Geometry: final body of the model. Coordinates: model frame, mm. Face numbers are marked on the shaded views. A direction names the side the tool comes from. Give positions to 0.01 mm unless a question says otherwise; leave off trailing zeros. Write each loop counter-clockwise with the first axis right and the second up, starting at its lowest first coordinate (ties: lowest second). Pieces come first, ordered by that corner, then holes. Notation, with made-up numbers: (-9.75, 10) - (-5.75, 10) arc R6 cw to (-5.75, 15) - close; hole circle Ø1 at (-6.75, -30). An arc over 180 degrees is marked (long way). One line per question, with ' | ' between items. Start each with the question number.
```python
from build123d import *

# Parameters (mm, degrees)
SALIENTE_EXTRUIR1_DEPTH           = 2
SALIENTE_EXTRUIR4_DEPTH           = 28
CROQUIS6_W                        = 6.2
CROQUIS6_H                        = 25
CORTAR_EXTRUIR2_DEPTH             = 6.2
CORTAR_EXTRUIR3_REACH             = 24
CROQUIS7_R                        = 1.6
CORTAR_EXTRUIR4_REACH             = 25.8
CROQUIS8_R                        = 1.6
CORTAR_EXTRUIR5_DEPTH             = 16.8
CORTAR_EXTRUIR6_DEPTH             = 2.5
CORTAR_EXTRUIR6_DIRECTION_2_REACH = 19
CROQUIS11_W                       = 0.3
CROQUIS11_H                       = 13.87
CORTAR_EXTRUIR7_DEPTH             = 6.2
CORTAR_EXTRUIR8_REACH             = 8.5
CROQUIS12_R                       = 1.6
CORTAR_EXTRUIR9_DEPTH             = 3
CORTAR_EXTRUIR10_DEPTH            = 6.5


with BuildPart() as part:
    # Croquis1 → Saliente-Extruir1 (new body)
    with BuildSketch(Plane.XY):
        Polygon((0, 0), (0, -4), (11, -4), (17, -10), (17, -17), (24, -17), (24, 0), (15.5, 0), (9.5, 6), (9.5, 11.13), (6.5, 11.13), (6.5, 25), (0, 25), align=None)
    extrude(amount=SALIENTE_EXTRUIR1_DEPTH)

    # Croquis5 → Saliente-Extruir4 (add)
    with BuildSketch(Plane.XY.offset(2)):
        Polygon((22, -17), (22, -3.5), (24, -3.5), (24, 0), (15.5, 0), (9.5, 6), (9.5, 11.13), (6.5, 11.13), (6.5, 25), (0, 25), (0, -4), (11, -4), (17, -10), (17, -17), align=None)
    extrude(amount=SALIENTE_EXTRUIR4_DEPTH)

    # Croquis6 → Cortar-Extruir2 (cut)
    with BuildSketch(Plane.XY.offset(30)):
        with Locations((3.1, 12.5)):
            Rectangle(CROQUIS6_W, CROQUIS6_H)
    extrude(amount=-CORTAR_EXTRUIR2_DEPTH, mode=Mode.SUBTRACT)

    # Croquis7 → Cortar-Extruir3 (cut, up to next)
    with BuildSketch(Plane(origin=(22, 0, 0), x_dir=(0, 0, -1), z_dir=(1, 0, 0)), mode=Mode.PRIVATE) as cortar_extruir3_sk1:
        with Locations((-18.55, -6.05)):
            Circle(CROQUIS7_R)
    cortar_extruir3_tool1 = extrude(cortar_extruir3_sk1.sketch, amount=-CORTAR_EXTRUIR3_REACH, mode=Mode.PRIVATE) & part.part
    add(cortar_extruir3_tool1.solids().sort_by_distance((22, -6.05, 18.55))[0], mode=Mode.SUBTRACT)
    # Croquis7 → Cortar-Extruir3 (cut, up to next)
    with BuildSketch(Plane(origin=(22, 0, 0), x_dir=(0, 0, -1), z_dir=(1, 0, 0)), mode=Mode.PRIVATE) as cortar_extruir3_sk2:
        with Locations((-6.45, -6.05)):
            Circle(CROQUIS7_R)
    cortar_extruir3_tool2 = extrude(cortar_extruir3_sk2.sketch, amount=-CORTAR_EXTRUIR3_REACH, mode=Mode.PRIVATE) & part.part
    add(cortar_extruir3_tool2.solids().sort_by_distance((22, -6.05, 6.45))[0], mode=Mode.SUBTRACT)

    # Croquis8 → Cortar-Extruir4 (cut, up to next)
    with BuildSketch(Plane.XY.offset(23.8), mode=Mode.PRIVATE) as cortar_extruir4_sk1:
        with Locations((3.1, 4)):
            Circle(CROQUIS8_R)
    cortar_extruir4_tool1 = extrude(cortar_extruir4_sk1.sketch, amount=-CORTAR_EXTRUIR4_REACH, mode=Mode.PRIVATE) & part.part
    add(cortar_extruir4_tool1.solids().sort_by_distance((3.1, 4, 23.8))[0], mode=Mode.SUBTRACT)

    # Croquis9 → Cortar-Extruir5 (cut)
    with BuildSketch(Plane(origin=(0, 0, 0), x_dir=(-1, 0, 0), z_dir=(0, 0, -1))):
        Polygon((-5.95, 2.354551733), (-3.1, 0.709103466), (-0.25, 2.354551733), (-0.25, 5.645448267), (-3.1, 7.290896534), (-5.95, 5.645448267), align=None)
    extrude(amount=-CORTAR_EXTRUIR5_DEPTH, mode=Mode.SUBTRACT)

    # Croquis10 → Cortar-Extruir6 (cut)
    with BuildSketch(Plane.ZY.offset(-17)):
        Polygon((3.159103466, -6.05), (4.804551733, -8.9), (8.095448267, -8.9), (9.740896534, -6.05), (8.095448267, -3.2), (4.804551733, -3.2), align=None)
        Polygon((15.259103466, -6.05), (16.904551733, -8.9), (20.195448267, -8.9), (21.840896534, -6.05), (20.195448267, -3.2), (16.904551733, -3.2), align=None)
    extrude(amount=-CORTAR_EXTRUIR6_DEPTH, mode=Mode.SUBTRACT)

    # Croquis10 → Cortar-Extruir6 direction 2 (cut, up to next)
    with BuildSketch(Plane.ZY.offset(-17), mode=Mode.PRIVATE) as cortar_extruir6_direction_2_sk1:
        Polygon((3.159103466, -6.05), (4.804551733, -8.9), (8.095448267, -8.9), (9.740896534, -6.05), (8.095448267, -3.2), (4.804551733, -3.2), align=None)
    cortar_extruir6_direction_2_tool1 = extrude(cortar_extruir6_direction_2_sk1.sketch, amount=CORTAR_EXTRUIR6_DIRECTION_2_REACH, mode=Mode.PRIVATE) & part.part
    add(cortar_extruir6_direction_2_tool1.solids().sort_by_distance((17, -6.05, 6.45))[0], mode=Mode.SUBTRACT)
    # Croquis10 → Cortar-Extruir6 direction 2 (cut, up to next)
    with BuildSketch(Plane.ZY.offset(-17), mode=Mode.PRIVATE) as cortar_extruir6_direction_2_sk2:
        Polygon((15.259103466, -6.05), (16.904551733, -8.9), (20.195448267, -8.9), (21.840896534, -6.05), (20.195448267, -3.2), (16.904551733, -3.2), align=None)
    cortar_extruir6_direction_2_tool2 = extrude(cortar_extruir6_direction_2_sk2.sketch, amount=CORTAR_EXTRUIR6_DIRECTION_2_REACH, mode=Mode.PRIVATE) & part.part
    add(cortar_extruir6_direction_2_tool2.solids().sort_by_distance((17, -6.05, 18.55))[0], mode=Mode.SUBTRACT)

    # Croquis11 → Cortar-Extruir7 (cut)
    with BuildSketch(Plane.XY.offset(30)):
        with Locations((6.35, 18.065)):
            Rectangle(CROQUIS11_W, CROQUIS11_H)
    extrude(amount=-CORTAR_EXTRUIR7_DEPTH, mode=Mode.SUBTRACT)

    # Croquis12 → Cortar-Extruir8 (cut, up to next)
    with BuildSketch(Plane(origin=(6.5, 0, 0), x_dir=(0, 0, -1), z_dir=(1, 0, 0)), mode=Mode.PRIVATE) as cortar_extruir8_sk1:
        with Locations((-9.2, 15.3)):
            Circle(CROQUIS12_R)
    cortar_extruir8_tool1 = extrude(cortar_extruir8_sk1.sketch, amount=-CORTAR_EXTRUIR8_REACH, mode=Mode.PRIVATE) & part.part
    add(cortar_extruir8_tool1.solids().sort_by_distance((6.5, 15.3, 9.2))[0], mode=Mode.SUBTRACT)

    # Croquis13 → Cortar-Extruir9 (cut)
    with BuildSketch(Plane.ZY):
        Polygon((9.2, 18.590896534), (6.35, 16.945448267), (6.35, 13.654551733), (9.2, 12.009103466), (12.05, 13.654551733), (12.05, 16.945448267), align=None)
    extrude(amount=-CORTAR_EXTRUIR9_DEPTH, mode=Mode.SUBTRACT)

    # Croquis14 → Cortar-Extruir10 (cut)
    with BuildSketch(Plane.XY.offset(30)):
        Polygon((15.5, 0), (15.5, -4), (11, -4), (17, -10), (17, -17), (22, -17), (22, -3.5), (24, -3.5), (24, 0), align=None)
    extrude(amount=-CORTAR_EXTRUIR10_DEPTH, mode=Mode.SUBTRACT)


solid = part.part
```
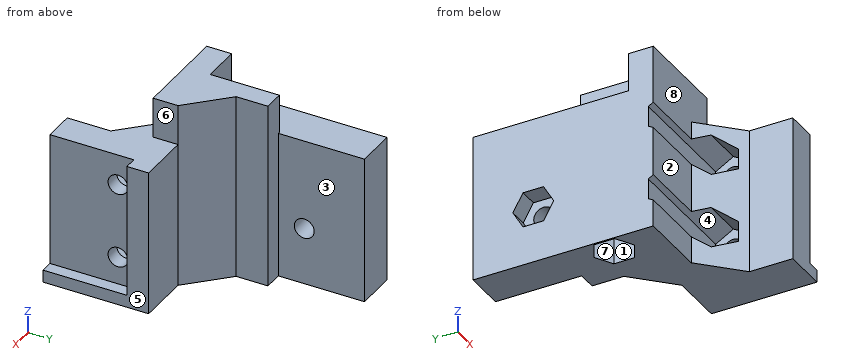
1) Section A-A, the plane z = 18.55. Output: boundary loops of the cut face in (x, y), plus the area to 3 significant figures.
2) Reachability of the marked faces 1, 2, 3, 4 and 5 from +Z, -Z, +X, -X, +Y, -Y: full face, straight path, thin tool, end or side. Return the list, or none.
3) Pull-direction query (X, two-part tool) for the marked faces 6, 7 and 8; classes: +X half, -X half, draft (parallel to the pull), parting line (faces both ways), or undercut.
4) First-contact query: pin 1 Ø7 at (x, y) = (5, 18.5) entering from +Z; pin 2 Ø1.6 at (x, z) = (17.5, 18.5) entering from +Y; pin 3 Ø7 at (y, z) = (-8.5, 17) entering from +X; pin 4 Ø10 at (x, y) = (17, 17) entering from +Z. Flat tips, straight axial feed; report the tip coordinate or a pass-through.
5) Line query: L1, parallel to Y at x = 5.5, z = 9.25; L2, parallel to Y at x = 4.5, z = 9.2; L3, parallel to Y at x = 20.3, z = 18.55. Output: solid intervals per line, ascending.
6) Section D-D, the plane y = 15.3. Output: boundary loops of the cut face in (x, z).
7) Section B-B, the plane y = 4. Output: boundary loops of the cut face in (x, z).
8) Section C-C, the plane x = 18.5. Output: boundary loops of the cut face in (y, z), plus the area to 3 significant figures.
Answer key:
1) outline: (0, -3.2) - (19.5, -3.2) - (19.5, -4.45) - (22, -4.45) - (22, -3.5) - (24, -3.5) - (24, 0) - (15.5, 0) - (9.5, 6) - (9.5, 11.13) - (6.5, 11.13) - (6.5, 25) - (0, 25) - close; (15.9, -8.9) - (17, -10) - (17, -17) - (22, -17) - (22, -7.65) - (19.5, -7.65) - (19.5, -8.9) - close; hole circle Ø3.2 at (3.1, 4) | area: 331 mm^2
2) face 1: -Z | face 2: +Z, -Z, -X, -Y | face 3: +Z, -Z, +X, +Y | face 4: -X | face 5: +Z, -Z, +X, +Y, -Y
3) face 6: +X half | face 7: undercut | face 8: draft
4) pin 1: z = 23.8 | pin 2: y = 0 | pin 3: x = 22 | pin 4: through
5) L1: -4 to 2.09, 5.91 to 13.7, 16.9 to 25 | L2: -4 to 1.52, 6.48 to 13.7, 16.9 to 25 | L3: -17 to -7.65, -4.45 to 0
6) outline: (0, 0) - (6.5, 0) - (6.5, 7.6) - (3, 7.6) - (3, 6.35) - (0, 6.35) - close; (0, 12.05) - (3, 12.05) - (3, 10.8) - (6.5, 10.8) - (6.5, 23.8) - (0, 23.8) - close
7) outline: (0, 0) - (0.25, 0) - (0.25, 16.8) - (1.5, 16.8) - (1.5, 23.8) - (0, 23.8) - close; (4.7, 16.8) - (5.95, 16.8) - (5.95, 0) - (11.5, 0) - (11.5, 30) - (6.2, 30) - (6.2, 23.8) - (4.7, 23.8) - close
8) outline: (-17, 0) - (0, 0) - (0, 23.5) - (-17, 23.5) - close; hole (-8.9, 4.8) - (-6.05, 3.16) - (-3.2, 4.8) - (-3.2, 8.1) - (-6.05, 9.74) - (-8.9, 8.1) - close; hole (-8.9, 16.9) - (-6.05, 15.26) - (-3.2, 16.9) - (-3.2, 20.2) - (-6.05, 21.84) - (-8.9, 20.2) - close | area: 343 mm^2
